The listing builds one solid part. Answer for the finished solid, in the listing's coordinates (mm). Face numbers are marked on the shaded views. Round coordinates to 2 decimals unless told otherwise and drop trailing zeros. Write each loop counter-clockwise with the first axis right and the second up, starting at its lowest first coordinate (ties: lowest second). Pieces come first, ordered by that corner, then holes. Notation, with made-up numbers: (-21, 17.25) - (35, 17.25) arc R11 cw to (35, 27.25) - close; hole circle Ø3 at (72, 31.25). An arc over 180 degrees is marked (long way). Answer as CSV lines item,"result". Start each with the question number.
Item 1: Flat-ended cylindrical pins translate along their axes: pin 1 (4.5 mm diameter, centred on x = 24, z = 3, fed in from +Y); pin 2 (4 mm diameter, centred on x = -128.54, z = -3.96, fed in from +Y). Find the tip coordinate at first contact, or state that the pin passes through.
Item 2: A cutting plane is placed at B-B on y = 1.7. Determine the outline of the cut face in (x, z).
Item 3: A cutting plane is placed at A-A on x = -111. Determine the outline of the cut face in (y, z), and give its area (3 significant figures).
Item 4: For a pull along X with two mould halves and no side action, classify the marked faces 1 and 2 as pulls with the +X half, pulls with the -X half, needs draft (parallel to the pull), parting line crosses it, or undercut.
Item 5: Straight lines are drawn through the part: line 1 along X through (y, z) = (0.5, 3.25); line 2 along X through (y, z) = (0.75, -4); line 3 along X through (y, z) = (1.9, 4). For each, find the intervals that lie inside material, in ascending order. Write a range as [from, to].
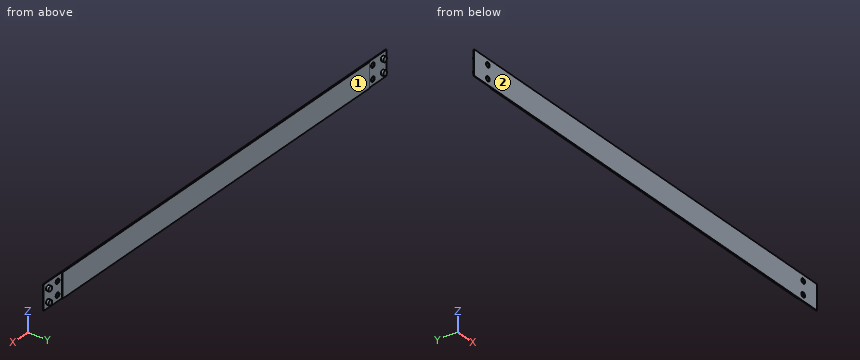
Autodesk Fusion 360 part; units mm, degrees
sketch "Sketch1" plane through (0, 0, 0) normal (0, 1, 0) x (1, 0, 0)
  line L0 (140, -7.5) -> (-140, -7.5)
  line L1 (-140, -7.5) -> (-140, 7.5)
  line L2 (-140, 7.5) -> (140, 7.5)
  line L3 (140, 7.5) -> (140, -7.5)
  line L4 (140, -7.5) -> (-140, 7.5) construction
  line L5 (-140, -7.5) -> (140, 7.5) construction
  line L6 (-125, 7.5) -> (-125, -7.5)
  line L7 (-140, 7.5) -> (-125, -7.5) construction
  line L8 (-125, 7.5) -> (-140, -7.5) construction
  circle A0 centre (-136.4645, 3.9645) radius 1.5
  circle A1 centre (-128.5355, 3.9645) radius 1.5
  line L9 (1.75, 0) -> (22.5, 0)
  circle A2 centre (-136.4645, -3.9645) radius 1.5
  circle A3 centre (-128.5355, -3.9645) radius 1.5
  line L10 (0, -20) -> (0, -2.5)
  line L11 (125, 7.5) -> (125, -7.5)
  circle A4 centre (128.5355, 3.9645) radius 1.5
  circle A5 centre (128.5355, -3.9645) radius 1.5
  circle A6 centre (136.4645, -3.9645) radius 1.5
  circle A7 centre (136.4645, 3.9645) radius 1.5
  dimension "d1" = 280
  dimension "d2" = 15
  dimension "d3" = 15
  dimension "d4" = 3
  dimension "d5" = 3
  dimension "d6" = 5
  dimension "d7" = 5
extrude "Extrude1" add sketch "Sketch1" along normal blind 0.9 contours L0 L2 L6 L11
extrude "Extrude2" add sketch "Sketch1" along normal blind 0.45 contours L0 L2 L3 L11 | L0 L1 L2 L6
extrude "Extrude3" add sketch "Sketch1" along normal blind 2 contours A0 | A2 | A6 | A7
move_face "OffsetFaces1" offset -0.2 2 faces at (140, 0.15, -2.5) (-140, 0.15, 2.5)
Geometry says:
1,pin 1,"stops at y = 0.9"
1,pin 2,"stops at y = 0.45"
2,outline,"circle Ø3 at (-136.46, -3.96); circle Ø3 at (-136.46, 3.96); circle Ø3 at (136.46, -3.96); circle Ø3 at (136.46, 3.96)"
3,outline,"(0, -7.5) - (0.9, -7.5) - (0.9, 7.5) - (0, 7.5) - close"
3,area,"13.5 mm^2"
4,face 1,"undercut"
4,face 2,"needs draft"
5,line 1,"x = [-137.78, -135.15], [-125, 125], [135.15, 137.78]"
5,line 2,"x = [-137.96, -134.96], [-125, 125], [134.96, 137.96]"
5,line 3,"x = [-137.96, -134.96], [134.96, 137.96]"
